Geometry: final body of the model. Coordinates: model frame, mm. A direction names the side the tool comes from. Coordinates: 2 decimals unless noted, no trailing zeros. Loops run counter-clockwise (first coordinate to the right, second up) from the corner with the lowest first, then second, coordinate; pieces in that order, holes last. Notation, with made-up numbers: (6.25, 84.25) - (13.25, 84.25) arc R31 cw to (13.25, 115.25) - close; hole circle Ø9 at (-37, 9). An arc over 180 degrees is marked (long way). Answer in a Markdown table with one row per item.
from build123d import *

# Parameters (mm, degrees)
SKIZZE1_R                       = 1.75
AUFSATZ_LINEAR_AUSTRAGEN1_DEPTH = 12
SKIZZE1_4_W                     = 12
SKIZZE1_4_H                     = 55
SKIZZE1_4_W_2                   = 150
SKIZZE1_4_H_2                   = 12
SCHNITT_LINEAR_AUSTRAGEN2_DEPTH = 4
VERRUNDUNG1_R                   = 3


with BuildPart() as part:
    # Skizze1 → Aufsatz-Linear austragen1 (new body)
    with BuildSketch(Plane.XY):
        with BuildLine():
            Line((24.14, 88), (49.14, 88))
            add(Edge.make_bspline(
                [(49.14, 88), (47.999428855, 47.699903884), (75, 12.5)],
                knots=[0, 0, 0, 1, 1, 1], degree=2))
            Line((75, 12.5), (75, -41))
            Line((75, -41), (-75, -41))
            Line((-75, -41), (-75, 12.5))
            add(Edge.make_bspline(
                [(24.14, 88), (26.807525043, 22.962561466), (-75, 12.5)],
                knots=[0, 0, 0, 1, 1, 1], degree=2))
        make_face()
        with Locations((-50, 0)):
            Circle(SKIZZE1_R, mode=Mode.SUBTRACT)
        Circle(SKIZZE1_R, mode=Mode.SUBTRACT)
        with Locations((50, 0)):
            Circle(SKIZZE1_R, mode=Mode.SUBTRACT)
        with Locations((36.64, 69)):
            Circle(SKIZZE1_R, mode=Mode.SUBTRACT)
        with Locations((36.64, 39)):
            Circle(SKIZZE1_R, mode=Mode.SUBTRACT)
    extrude(amount=AUFSATZ_LINEAR_AUSTRAGEN1_DEPTH)

    # Skizze1_4 → Schnitt-Linear austragen2 (cut)
    with BuildSketch(Plane.XY):
        with Locations((36.64, 54)):
            Rectangle(SKIZZE1_4_W, SKIZZE1_4_H)
        Rectangle(SKIZZE1_4_W_2, SKIZZE1_4_H_2)
    extrude(amount=SCHNITT_LINEAR_AUSTRAGEN2_DEPTH, mode=Mode.SUBTRACT)

    # Verrundung1
    verrundung1_edges = [part.edges().sort_by_distance(p)[0] for p in [
        (75, -41, 6),
        (75, 12.5, 6),
        (49.14, 88, 6),
        (-75, -41, 6),
        (-75, 12.5, 6),
        (24.14, 88, 6),
    ]]
    fillet(verrundung1_edges, radius=VERRUNDUNG1_R)


solid = part.part
(1) Cut plane A-A on y = 0. Output: boundary loops of the cut face in (x, z).
Verdict:
| item | result |
|---|---|
| outline | (-75, 4) - (-51.75, 4) - (-51.75, 12) - (-75, 12) - close; (-48.25, 4) - (-1.75, 4) - (-1.75, 12) - (-48.25, 12) - close; (1.75, 4) - (48.25, 4) - (48.25, 12) - (1.75, 12) - close; (51.75, 4) - (75, 4) - (75, 12) - (51.75, 12) - close |
(2) Cut plane B-B on x = 36.64. Output: boundary loops of the cut face in (y, z), then the cut area to 3 significant figures.
Verdict:
| item | result |
|---|---|
| outline | (-41, 0) - (-6, 0) - (-6, 4) - (6, 4) - (6, 0) - (26.5, 0) - (26.5, 4) - (37.25, 4) - (37.25, 12) - (-41, 12) - close; (40.75, 4) - (67.25, 4) - (67.25, 12) - (40.75, 12) - close; (70.75, 4) - (81.5, 4) - (81.5, 0) - (88, 0) - (88, 12) - (70.75, 12) - close |
| area | 1,220 mm² |
(3) Access query for faces 5 (the face through (37, 54, 4)), 6 (the face through (-1, -6, 2)), 7 (the face through (75, -13, 6)). Directions: +Z, -Z, +X, -X, +Y, -Y. A direction counts if a zero-diameter tool reaches every point of the face in a straight line with its end or side. Return the directions, or none.
Verdict:
| item | result |
|---|---|
| face 5 | -Z |
| face 6 | -Z, +X, -X |
| face 7 | +Z, -Z, +X, +Y, -Y |
(4) Ray query, probe 1 along X at (y, z) = (0, 8.75); probe 2 along Y at (x, z) = (1.5, 3); probe 3 along Y at (x, z) = (-14.5, 0.75). Return the intervals inside material, ascending.
Verdict:
| item | result |
|---|---|
| probe 1 | x = -75 to -51.75, -48.25 to -1.75, 1.75 to 48.25, 51.75 to 75 |
| probe 2 | y = -41 to -6, 6 to 37.23 |
| probe 3 | y = -41 to -6, 6 to 27.46 |
(5) Cut plane C-C on z = 2.25. State how many separate pieces and enclosed holes the cut face has, then the cut area to 3 significant figures.
Verdict:
| item | result |
|---|---|
| separate pieces | 2 |
| enclosed holes | 1 |
| area | 9,570 mm² |
(6) Pull-direction query (X, two-part tool) for faces 1 (the face through (74.14, -40.1, 6.08)), 2 (the face through (37, 26.5, 2)), 3 (the face through (1, -23, 0)), 4 (the face through (-75, -14, 6)); classes: pulls with the +X half, pulls with the -X half, needs draft (parallel to the pull), parting line crosses it, or undercut.
Verdict:
| item | result |
|---|---|
| face 1 | pulls with the +X half |
| face 2 | undercut |
| face 3 | needs draft |
| face 4 | pulls with the -X half |
(7) First-contact query: pin 1 Ø5.5 at (x, y) = (36.64, 39) entering from -Z; pin 2 Ø2 at (x, y) = (-50, 0) entering from -Z; pin 3 Ø3 at (x, z) = (-33.5, 1) entering from +Y; pin 4 Ø4.5 at (y, z) = (43.5, 2.5) entering from +X. Flat tips, straight axial feed; report the tip coordinate or a pass-through.
Verdict:
| item | result |
|---|---|
| pin 1 | stops at z = 4 |
| pin 2 | passes through |
| pin 3 | stops at y = 20.71 |
| pin 4 | stops at x = 58 |
